from build123d import *

# Parameters (mm, degrees)
BOSS_EXTRUDE1_DEPTH = 12.7
SKETCH2_R           = 1.5875
CUT_EXTRUDE1_DEPTH  = 32.75


with BuildPart() as part:
    # Sketch1 → Boss-Extrude1 (new body)
    with BuildSketch(Plane(origin=(0, 0, 0), x_dir=(1, 0, 0), z_dir=(0, 1, 0))):
        Polygon((0, 9.525), (-12.7, 9.525), (-12.7, 15.875), (6.35, 15.875), (6.35, 6.35), (37.410945752, 6.35), (37.410945752, 15.875), (56.460945752, 15.875), (56.460945752, 9.525), (43.760945752, 9.525), (43.760945752, -9.525), (56.460945752, -9.525), (56.460945752, -15.875), (37.410945752, -15.875), (37.410945752, -6.35), (6.35, -6.35), (6.35, -15.875), (-12.7, -15.875), (-12.7, -9.525), (0, -9.525), align=None)
    extrude(amount=BOSS_EXTRUDE1_DEPTH)

    # Sketch2 → Cut-Extrude1 (cut, through all)
    with BuildSketch(Plane.XY.offset(15.875)):
        with Locations((50.110945752, 6.35)):
            Circle(SKETCH2_R)
        with Locations((-6.35, 6.35)):
            Circle(SKETCH2_R)
    extrude(amount=-CUT_EXTRUDE1_DEPTH, mode=Mode.SUBTRACT)


solid = part.part
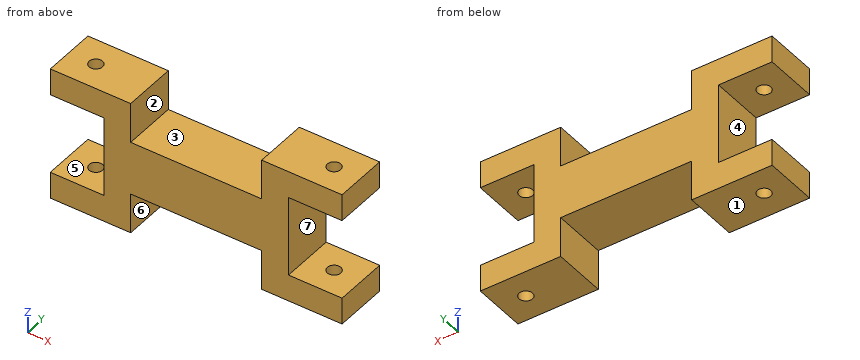
Could you check a few things on this model? Use its own coordinates, in mm. Face numbers are marked on the shaded views. A direction names the side the tool comes from. Give positions to 0.01 mm unless a question says otherwise; leave off trailing zeros. Write each loop counter-clockwise with the first axis right and the second up, starting at its lowest first coordinate (ties: lowest second). Pieces come first, ordered by that corner, then holes. Notation, with made-up numbers: (37, 62) -> (83, 62) arc R24 cw to (83, 85) -> close; hole circle Ø1 at (82.5, -40). An arc over 180 degrees is marked (long way). Answer as CSV lines item,"result". Start each with the question number.
(1) Please list where these lines run through material, in increasing order: line 1 (X direction, y = 7.75, z = -9); line 2 (Z direction, x = -7.5, y = 4) (3 decimals); line 3 (Y direction, x = -6.35, z = -13.5).
(2) I'm going to push flat-ended pins straight in: pin 1 Ø2 at (y, z) = (8, -1.5) entering from +X; pin 2 Ø1.5 at (x, y) = (21.5, 8.5) entering from -Z; pin 3 Ø6.5 at (x, y) = (15, 7.5) entering from +Z. Where does each tip first touch, or does it pass through?
(3) If we section it at A-A, the plane z = 11: Give the number of separate pieces and of enclosed holes in the cut face, and give its area (3 significant figures).
(4) Which directions (+Z, -Z, +X, -X, +Y, -Y) give clear straight access to the entire face, cutting with the end or side of a thin tool? Please do the marked faces 5, 6 and 7.
(5) If we section it at B-B, the plane x = -6.35: Write out the boundary of the cut face in (y, z) (1 decimal), and give its area (3 significant figures).
(6) If we section it at C-C, the plane y = 3: Write out the boundary of the cut face in (x, z) (3 decimals).
(7) If we mould it in two halves opening along X, with no side actions, what happens to the marked faces 1, 2, 3 and 4? For each: +X half, -X half, draft (parallel to the pull), parting line (faces both ways), or undercut.
Answer list:
1,line 1,"0 to 6.35, 37.41 to 43.76"
1,line 2,"-15.875 to -9.525, 9.525 to 15.875"
1,line 3,"0 to 4.76, 7.94 to 12.7"
2,pin 1,"x = 43.76"
2,pin 2,"z = -6.35"
2,pin 3,"z = 6.35"
3,separate pieces,"2"
3,enclosed holes,"2"
3,area,"468 mm^2"
4,face 5,"-X, +Y, -Y"
4,face 6,"-Z, +Y, -Y"
4,face 7,"+X, +Y, -Y"
5,outline,"(0, -15.9) -> (4.8, -15.9) -> (4.8, -9.5) -> (0, -9.5) -> close; (0, 9.5) -> (4.8, 9.5) -> (4.8, 15.9) -> (0, 15.9) -> close; (7.9, -15.9) -> (12.7, -15.9) -> (12.7, -9.5) -> (7.9, -9.5) -> close; (7.9, 9.5) -> (12.7, 9.5) -> (12.7, 15.9) -> (7.9, 15.9) -> close"
5,area,"121 mm^2"
6,outline,"(-12.7, -15.875) -> (6.35, -15.875) -> (6.35, -6.35) -> (37.411, -6.35) -> (37.411, -15.875) -> (56.461, -15.875) -> (56.461, -9.525) -> (43.761, -9.525) -> (43.761, 9.525) -> (56.461, 9.525) -> (56.461, 15.875) -> (37.411, 15.875) -> (37.411, 6.35) -> (6.35, 6.35) -> (6.35, 15.875) -> (-12.7, 15.875) -> (-12.7, 9.525) -> (0, 9.525) -> (0, -9.525) -> (-12.7, -9.525) -> close"
7,face 1,"draft"
7,face 2,"undercut"
7,face 3,"undercut"
7,face 4,"-X half"
